Autodesk Inventor part; units mm, degrees
ref_plane "Work Plane1" through (298.1208, 0, 0) normal (0, 1, 0) x (-1, 0, 0)
ref_plane "YZ Plane" through (0, 0, 0) normal (1, 0, 0) x (0, 1, 0)
ref_plane "XZ Plane" through (0, 0, 0) normal (0, 1, 0) x (-1, 0, 0)
sketch "Sketch1" plane through (0, 0, 0) normal (0, 0, 1) x (1, 0, 0)
  line L0 (0, 0) -> (26, 0)
  line L1 (0, 0) -> (0, 105)
  line L2 (0, 105) -> (26, 105)
  line L3 (26, 105) -> (26, 0)
  line L4 (0, 126) -> (0, -21)
  line L5 (-5.2, 0) -> (31.2, 0)
  dimension "d1" = 210
  dimension "d2" = 26
revolve "Body" add sketch "Sketch1" angle 360 about axis through (0, 0, 0) along (1, 0, 0)
sketch "Sketch2" plane through (0, 0, 0) normal (-1, 0, 0) x (0, 0, 1)
  circle A0 centre (0, 0) radius 105
  point P0 (0, 0)
hole "Thread" at (0, 0, 0) direction (1, 0, 0) diameter 161.7524 end through all
chamfer "Chamfer1" distance 8.5 angle 30 1 edges at (0, -105, 0) measured on face at (0, 48.5251, -83.6903)
sketch "Sketch3" plane through (26, 0, 0) normal (1, 0, 0) x (0, 0, -1)
  circle A0 centre (0, 0) radius 105
  line L0 (-8, 104.6948) -> (-8, 98)
  line L1 (-8, 98) -> (8, 98)
  line L2 (8, 98) -> (8, 104.6948)
  line L3 (0, -147) -> (0, 147)
  line L4 (-147, 0) -> (147, 0)
  dimension "d12" = 8
  dimension "d13" = 8
  dimension "d14" = 98
extrude "Groove1" cut sketch "Sketch3" against normal through all contours L2 L1 L3 A0 | L3 L1 L0 A0
pattern_circular "Grooves1" count 4 over 360 about axis through (-10, 0, 0) along (1, 0, 0) of "Groove1"
fillet "Fillet1" radius 2.6 4 edges at (26, 74.2462, 74.2462) (26, 74.2462, -74.2462) (26, -74.2462, -74.2462) (26, -74.2462, 74.2462)
chamfer "Chamfer2" distance 4.125 angle 45 1 edges at (26, 0, -80.8762) measured on face at (26, -86.7774, -38.7468)
chamfer "Chamfer3" distance 4.125 angle 45 1 edges at (0, 0, -80.8762) measured on face at (0, 90.9647, -4.5778)
ref_plane "Work Plane1" through (298.1208, 0, 0) normal (0, 1, 0) x (-1, 0, 0)
equation "\"d1\" = SD2"
equation "\"d2\" = KOH"
equation "\"d12\" = 0.5 * SNB"
equation "\"d13\" = 0.5 * SNB"
equation "\"d14\" = 0.5 * SD2 - SNT"
equation "\"d10\" = -0.5 * LADI + 0.5 * SD2"
equation "\"d11\" = FAWI2"
equation "\"d40\" = -0.5 * LADI + 0.5 * SD2"
equation "\"d18\" = RR"
equation "\"d19\" = 0.025 * NND"
equation "\"d41\" = 0.025 * NND"
equation "\"d21\" = 0.025 * NND"
equation "\"d42\" = 0.025 * NND"
equation "\"NND\" = 165"
equation "\"KOH\" = 26"
equation "\"SD2\" = 210"
equation "\"SNB\" = 16"
equation "\"SNT\" = 7"
equation "\"LADI\" = 193"
equation "\"RR\" = 2.6"
equation "\"FAWI2\" = 30deg"
equation "\"GUL\" = 0.61345 * PTC"
equation "\"THREADDIA\" = 165"
equation "\"TOA\" = 30deg"
equation "\"PTC\" = 3"
equation "\"GAL\" = 0.61345 * PTC"
equation "\"GD1\" = THREADDIA - 1.2269 * PTC"
properties part number "DIN 981 - KM 33" material "Steel, Mild"
Geometry check sheet. Reference: the model listing, model coordinates, mm. A direction names the side the tool comes from. Coordinates: 2 decimals unless noted, no trailing zeros. Order: outer loops, then holes, each group sorted by start corner. A loop starts at its lowest first (then second) coordinate and runs counter-clockwise, first axis right, second up. Notation, with made-up numbers: M 60.5,59 L 67.5,59 A13 ccw 67.5,76 Z; hole C -39.5,0 d5. An arc over 180 degrees is marked long. One line per question, with ' | ' between items. Start each with the question number.
Item 1: Material ranges on L1, parallel to Z at x = 18.25, y = 0; L2, parallel to Y at x = 21.5, z = -56, recorded low to high. Write a range as [from, to].
Item 2: Cross-section at B-B on x = 9. Enter the section's corners in (y, z), then the cut area to 3 significant figures.
Item 3: Draft check along Y on faces 1 (the cylindrical face through (14.283, -73.505, 74.98)), 2 (the flat face through (14, -101, 8)), 3 (the cylindrical face through (13.124, -80.188, -10.528)). Enter one of: pulls with the +Y half, pulls with the -Y half, needs draft (parallel to the pull), parting line crosses it, or undercut.
Item 4: Cross-section at A-A on z = 0. Enter the section's corners in (x, y) (3 decimals), then the cut area to 3 significant figures.
Item 5: Gauge pin test, flat ends, axial feed: pin 1 (6 mm diameter, centred on x = 22, y = -13, fed in from -Z); pin 2 (13 mm diameter, centred on x = 15, y = 0, fed in from +Z); pin 3 (6 mm diameter, centred on x = 14.5, z = 11.5, fed in from +Y). Record the tip position at first contact, or that the pin passes through.
Item 6: Set-up check for faces 4 (the flat face through (14, 101, -8)), 5 (the flat face through (14, -8, 101)), 6 (the flat face through (14, -101, -8)): record each of +Z, -Z, +X, -X, +Y, -Y from which the full face is reachable in a straight line by a thin tool's end or side.
Findings:
1) L1: z = [-98, -80.88], [80.88, 98] | L2: y = [-88.82, -58.35], [58.35, 88.82]
2) outline: M -104.69,-8 A105 ccw -8,-104.69 L -8,-98 L 8,-98 L 8,-104.69 A105 ccw 104.69,-8 L 98,-8 L 98,8 L 104.69,8 A105 ccw 8,104.69 L 8,98 L -8,98 L -8,104.69 A105 ccw -104.69,8 L -98,8 L -98,-8 Z; hole C 0,0 d161.75 | area: 13,600 mm²
3) face 1: pulls with the -Y half | face 2: needs draft | face 3: undercut
4) outline: M 0,-96.5 L 0.866,-98 L 26,-98 L 26,-85.001 L 21.875,-80.876 L 4.125,-80.876 L 0,-85.001 Z; M 0,85.001 L 4.125,80.876 L 21.875,80.876 L 26,85.001 L 26,98 L 0.866,98 L 0,96.5 Z | area: 855 mm²
5) pin 1: stops at z = -104.52 | pin 2: stops at z = 98 | pin 3: stops at y = 104.66
6) face 4: +X, -X, +Y | face 5: +Z, +X, -X | face 6: +X, -X, -Y
